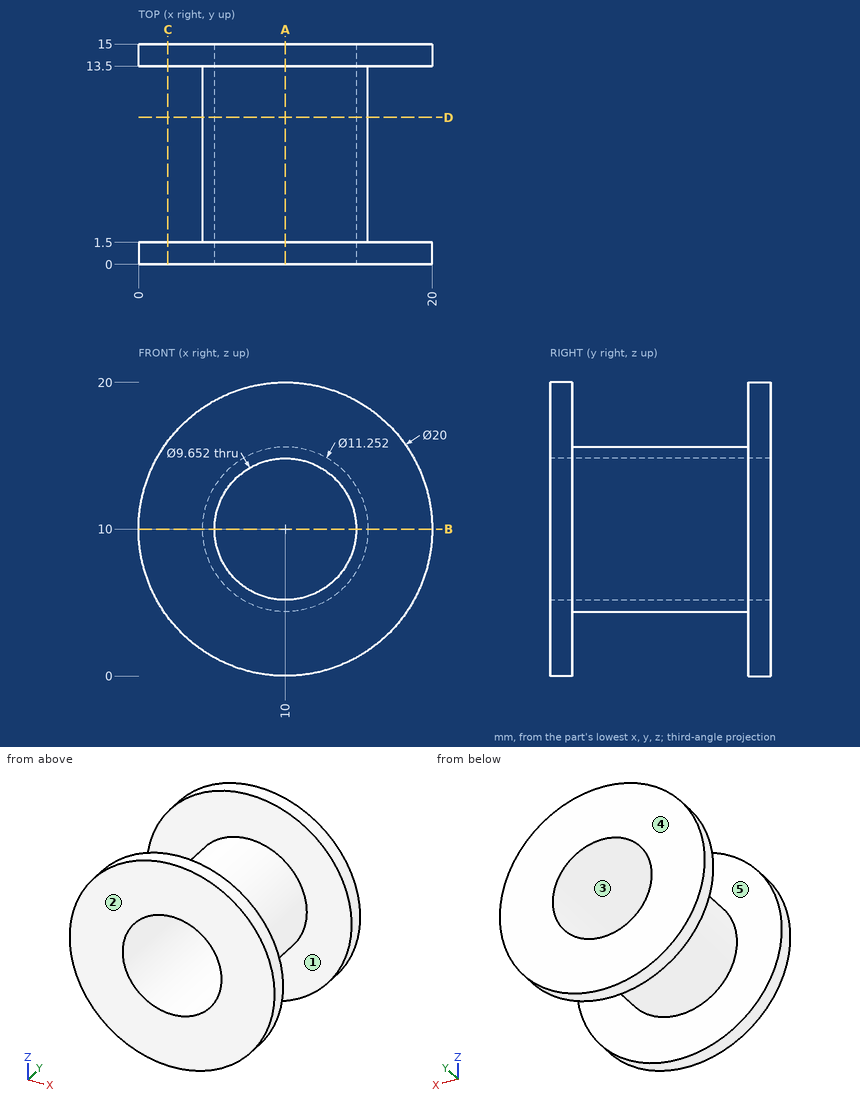
Geometry check sheet. Reference: drawing and pictorial views, mm from the part's lowest x, y, z. A direction names the side the tool comes from. Coordinates: 2 decimals unless noted, no trailing zeros. Order: outer loops, then holes, each group sorted by start corner. A loop starts at its lowest first (then second) coordinate and runs counter-clockwise, first axis right, second up. Notation, with made-up numbers: (40.25, 39.5) - (60.25, 39.5) arc R27 cw to (60.25, 68.5) - close; hole circle Ø11 at (81, 6). An arc over 180 degrees is marked (long way). Answer in a Markdown table with one row per item. Add a question column.
1) Cross-section at B-B, the plane z = 10. Record the cut outline in (x, y).
2) Material ranges on line 1 along Y through (x, z) = (13.25, 3.5); line 2 along X through (y, z) = (5, 10), recorded low to high. Write a range as [from, to].
3) Set-up check for the marked faces 1 and 2: record each of +Z, -Z, +X, -X, +Y, -Y from which the full face is reachable in a straight line by a thin tool's end or side.
4) Cross-section at D-D, the plane y = 10. Record the cut outline in (x, z).
5) Cross-section at A-A, the plane x = 10. Record the cut outline in (y, z), then the cut area to 3 significant figures.
6) Gauge pin test, flat ends, axial feed: P1, Ø8, axis at y = 11.5, z = 16, coming from the +X side; P2, Ø8, axis at y = 12.5, z = 5, coming from the +X side; P3, Ø3, axis at y = 11, z = 15.5, coming from the +X side. Record the tip position at first contact, or that the pin passes through.
7) Release check for a two-part mould opening along Y. For the marked faces 3, 4 and 5 record: +Y half, -Y half, draft (parallel to the pull), parting line (faces both ways), or undercut.
8) Cross-section at C-C, the plane x = 2. Record the cut outline in (y, z), then the cut area to 3 significant figures.
Check result:
| question | item | result |
|---|---|---|
| 1 | outline | (0, 0) - (5.17, 0) - (5.17, 15) - (0, 15) - (0, 13.5) - (4.37, 13.5) - (4.37, 1.5) - (0, 1.5) - close; (14.83, 0) - (20, 0) - (20, 1.5) - (15.63, 1.5) - (15.63, 13.5) - (20, 13.5) - (20, 15) - (14.83, 15) - close |
| 2 | line 1 | y = [0, 1.5], [13.5, 15] |
| 2 | line 2 | x = [4.37, 5.17], [14.83, 15.63] |
| 3 | face 1 | none |
| 3 | face 2 | +Z, -Z, +X, -X, -Y |
| 4 | outline | circle Ø11.25 at (10, 10); hole circle Ø9.65 at (10, 10) |
| 5 | outline | (0, 0) - (1.5, 0) - (1.5, 4.37) - (13.5, 4.37) - (13.5, 0) - (15, 0) - (15, 5.17) - (0, 5.17) - close; (0, 14.83) - (15, 14.83) - (15, 20) - (13.5, 20) - (13.5, 15.63) - (1.5, 15.63) - (1.5, 20) - (0, 20) - close |
| 5 | area | 50.2 mm² |
| 6 | P1 | stops at x = 19.67 |
| 6 | P2 | stops at x = 19.94 |
| 6 | P3 | stops at x = 13.96 |
| 7 | face 3 | draft |
| 7 | face 4 | +Y half |
| 7 | face 5 | undercut |
| 8 | outline | (0, 4) - (1.5, 4) - (1.5, 16) - (0, 16) - close; (13.5, 4) - (15, 4) - (15, 16) - (13.5, 16) - close |
| 8 | area | 36.0 mm² |
